Check sheet for the modelled part. Datum: model origin and axes. Units: mm. Face numbers are marked on the shaded views. A direction names the side the tool comes from. Give positions to 0.01 mm unless a question says otherwise; leave off trailing zeros. Order: outer loops, then holes, each group sorted by start corner. A loop starts at its lowest first (then second) coordinate and runs counter-clockwise, first axis right, second up.
Item 1: Access from +Z, -Z, +X, -X, +Y, -Y to the whole of each face (thin tool, end or side, straight path). Record for the marked faces 1, 2, 3 and 4.
Item 2: Gauge pin test, flat ends, axial feed: P1, Ø4, axis at x = -9, z = 12, coming from the +Y side; P2, Ø1.5, axis at x = 48, y = 7, coming from the +Z side; P3, Ø13, axis at x = -1, z = 28.5, coming from the -Y side. Record the tip position at first contact, or that the pin passes through.
Item 3: Material ranges on line 1 along Z through (x, y) = (-49.05, 13); line 2 along X through (y, z) = (19, 18); line 3 along Y through (x, z) = (-14.5, 10), recorded low to high.
Item 4: Sectioned sample at D-D on y = 6. Record the boundary of the cut face in (x, z).
Item 5: Sectioned sample at A-A on y = 13. Record the boundary of the cut face in (x, z).
Item 6: Sectioned sample at B-B on z = 23. Record the boundary of the cut face in (x, y), and give its area (3 significant figures).
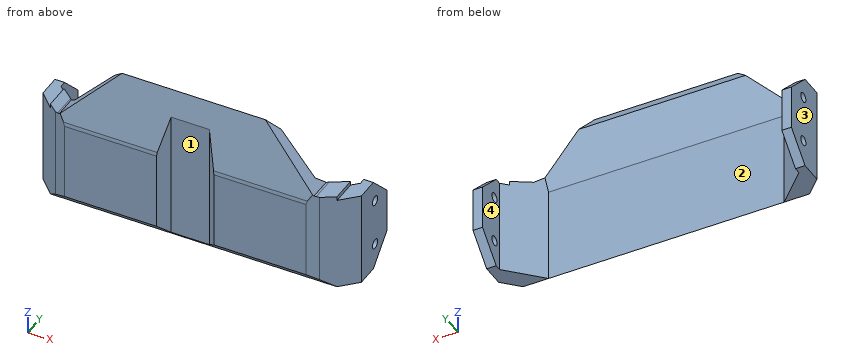
from build123d import *

# Parameters (mm, degrees)
F1_DEPTH      = 30
F2_SIZE       = 10
F4_DEPTH      = 50
F5_DEPTH      = 20
F6_DEPTH      = 25
F8_DEPTH      = 25.001
F9_DEPTH      = 25
F11_W         = 8
F11_H         = 3
F12_DEPTH     = 50.001
F13_T1_DEPTH  = 61.7168298797
F13_T3_DEPTH  = 40.0719817161
F13_T5_DEPTH  = 45.2357066129
F13_T10_DEPTH = 64.7177203375
F13_T15_DEPTH = 64.7177203375
F14_T1_DEPTH  = 56.7168298797
F14_T3_DEPTH  = 45.2357066129
F14_T5_DEPTH  = 35.0719817161
F15_R         = 1.5
F16_DEPTH     = 100.001
F18_SIZE      = 8
F19_SIZE      = 2.99999


# Not quite as in the source:
# - a fillet or chamfer that OpenCascade refuses, or shapes differently, is made with other operations: its cross-section is extruded or revolved along the edge and cut away or added
# - a fillet or chamfer is up to 0.001 mm smaller than in the source, because OpenCascade refuses the exact size


with BuildPart() as f1:
    # F0 (on Top) → F1 (new body)
    with BuildSketch(Plane.XY):
        Polygon((-47, 20), (-50, 20), (-50, -5), (50, -5), (50, 20), (47, 20), (47, 0), (-47, 0), align=None)
    extrude(amount=F1_DEPTH)

    # F2
    f2_edges = [f1.edges().sort_by_distance(p)[0] for p in [
        (-47, 0, 15),
        (47, 0, 15),
        (-50, -5, 15),
        (50, -5, 15),
    ]]
    chamfer(f2_edges, length=F2_SIZE)

    # F3 (on Right) → F4 (join, symmetric)
    with BuildSketch(Plane.YZ):
        Polygon((-5, 30), (0, 30), (2.9104275004, 49.2723931249), (0, 50), align=None)
    extrude(amount=F4_DEPTH, both=True)

    # F5 (add): faces of the model
    f5_faces = [f1.faces().sort_by_distance(p)[0] for p in [
        (46.0427350427, 7.6495726496, 30),
        (-46.0427350427, 7.6495726496, 30),
    ]]
    extrude(f5_faces, amount=F5_DEPTH)

    # F6 (cut): faces of the model
    f6_faces = [f1.faces().sort_by_distance(p)[0] for p in [
        (46.1111111111, -2.7777777778, 30),
        (-46.1111111111, -2.7777777778, 30),
    ]]
    extrude(f6_faces, amount=-F6_DEPTH, mode=Mode.SUBTRACT)

    # F7 (on face) → F8 (cut, through all)
    with BuildSketch(Plane.XZ.offset(5)):
        Polygon((40.5882352941, 32.3529411765), (45, 50), (37, 50), (22.5, 50), (40, 32.5), align=None)
        Polygon((45, 31.25), (45, 50), (40.5882352941, 32.3529411765), align=None)
        Polygon((45, 50), (47.9104275004, 49.2723931249), (45.1819017188, 31.2045245703), (50, 30), (50, 50), align=None)
    extrude(amount=-F8_DEPTH, mode=Mode.SUBTRACT)

    # F9 (cut): a face of the model
    f9_faces = [f1.faces().sort_by_distance(p)[0] for p in [
        (46.0411372728, 0, 41.900989059),
    ]]
    extrude(f9_faces, amount=-F9_DEPTH, mode=Mode.SUBTRACT)

    # F10: F1 across plane


with BuildPart() as f1_1:
    add(f1.part)
    add(f1.part.mirror(Plane.YZ), mode=Mode.INTERSECT)

    # F11 (on face) → F12 (cut, through all)
    with BuildSketch(Plane(origin=(0, 0, 0), x_dir=(1, 0, 0), z_dir=(0, 0, -1))):
        with Locations((0, 3.5)):
            Rectangle(F11_W, F11_H)
    extrude(amount=-F12_DEPTH, mode=Mode.SUBTRACT)

    # F13: chamfer of 5 on 5 edges, made by hand

    # F13_s2 → F13_t1 (cut)
    with BuildSketch(Plane.YZ.offset(-52.8584149398)):
        Polygon((0, 0), (-5, 5), (-5, 0), align=None)
    extrude(amount=F13_T1_DEPTH, mode=Mode.SUBTRACT)

    # F13_s4 → F13_t3 (cut)
    with BuildSketch(Plane.YZ.offset(-42.0359908581)):
        Polygon((-5, 29.3844718719), (-4.8507125007, 30.5971499971), (-5, 30), align=None)
    extrude(amount=F13_T3_DEPTH, mode=Mode.SUBTRACT)

    # F13_s6 → F13_t5 (cut)
    with BuildSketch(Plane.XY.offset(-5.6428543011)):
        Polygon((-41.4644660941, -3.5355339059), (-37.9289321881, -5), (-40, -5), align=None)
    extrude(amount=F13_T5_DEPTH, mode=Mode.SUBTRACT)


with BuildPart() as f13_tool8:
    # F13_s9 → F13_t10 (new body)
    with BuildSketch(Plane.XY.offset(-12.8584149398)):
        Polygon((9, -5), (4, 0), (4, -5), align=None)
    extrude(amount=F13_T10_DEPTH)

    split(bisect_by=Plane.XZ.offset(2), keep=Keep.TOP)


with BuildPart() as f1_2:
    add(f1_1.part)

    # F13_t7: cut F13_tool8
    add(f13_tool8.part, mode=Mode.SUBTRACT)


with BuildPart() as f13_tool13:
    # F13_s14 → F13_t15 (new body)
    with BuildSketch(Plane.XY.offset(-12.8584149398)):
        Polygon((-4, 0), (-9, -5), (-4, -5), align=None)
    extrude(amount=F13_T15_DEPTH)

    split(bisect_by=Plane.XZ.offset(2), keep=Keep.TOP)


with BuildPart() as f1_3:
    add(f1_2.part)

    # F13_t12: cut F13_tool13
    add(f13_tool13.part, mode=Mode.SUBTRACT)

    # F14: chamfer of 5 on 3 edges, made by hand

    # F14_s2 → F14_t1 (cut)
    with BuildSketch(Plane.YZ.offset(-3.8584149398)):
        Polygon((-5, 5), (0, 0), (-5, 0), align=None)
    extrude(amount=F14_T1_DEPTH, mode=Mode.SUBTRACT)

    # F14_s4 → F14_t3 (cut)
    with BuildSketch(Plane.XY.offset(-5.6428543011)):
        Polygon((41.4644660941, -3.5355339059), (37.9289321881, -5), (40, -5), align=None)
    extrude(amount=F14_T3_DEPTH, mode=Mode.SUBTRACT)

    # F14_s6 → F14_t5 (cut)
    with BuildSketch(Plane.YZ.offset(6.9640091419)):
        Polygon((-5, 29.3844718719), (-4.8507125007, 30.5971499971), (-5, 30), align=None)
    extrude(amount=F14_T5_DEPTH, mode=Mode.SUBTRACT)

    # F15 (on face) → F16 (cut, through all)
    with BuildSketch(Plane(origin=(-50, 0, 0), x_dir=(0, -1, 0), z_dir=(-1, 0, 0))):
        with Locations((-13, 23)):
            Circle(F15_R)
        with Locations((-13, 8)):
            Circle(F15_R)
    extrude(amount=-F16_DEPTH, mode=Mode.SUBTRACT)

    # F17: F1 across plane


with BuildPart() as f1_4:
    add(f1_3.part)
    add(f1_3.part.mirror(Plane.YZ), mode=Mode.INTERSECT)

    # F18
    f18_edges = [f1_4.edges().sort_by_distance(p)[0] for p in [
        (48.5, 20, 0),
        (-48.5, 20, 0),
        (-48.5, 20, 30),
        (48.5, 20, 30),
    ]]
    chamfer(f18_edges, length=F18_SIZE)

    # F19 (size 3 in the source; OpenCascade refuses exactly that, so slightly less here)
    f19_edges = [f1_4.edges().sort_by_distance(p)[0] for p in [
        (0, 2.910428, 49.272393),
    ]]
    chamfer(f19_edges, length=F19_SIZE)


solid = f1_4.part
Report:
1. face 1: +Z, -Z, -Y
1. face 2: -Z, +Y
1. face 3: +Z, -Z, -X, +Y, -Y
1. face 4: +Z, -Z, +Y
2. P1: stops at y = 0
2. P2: stops at z = 30
2. P3: stops at y = -3.5
3. line 1: z = 1 to 6.5, 9.5 to 21.5, 24.5 to 29
3. line 2: x = -50 to -47, 47 to 50
3. line 3: y = -5 to 0
4. outline: (-50, 0) - (-43, 0) - (-43, 31.75) - (-45, 31.25) - (-45, 30) - (-50, 30) - close; (43, 0) - (50, 0) - (50, 30) - (45, 30) - (45, 31.25) - (43, 31.75) - close
5. outline: (-50, 1) - (-47, 1) - (-47, 6.5) - (-50, 6.5) - close; (-50, 9.5) - (-47, 9.5) - (-47, 21.5) - (-50, 21.5) - close; (-50, 24.5) - (-47, 24.5) - (-47, 29) - (-50, 29) - close; (47, 1) - (50, 1) - (50, 6.5) - (47, 6.5) - close; (47, 9.5) - (50, 9.5) - (50, 21.5) - (47, 21.5) - close; (47, 24.5) - (50, 24.5) - (50, 29) - (47, 29) - close
6. outline: (-50, 5) - (-41.46, -3.54) - (-37.93, -5) - (-9, -5) - (-6, -2) - (6, -2) - (9, -5) - (37.93, -5) - (41.46, -3.54) - (50, 5) - (50, 11.5) - (47, 11.5) - (47, 10) - (37, 0) - (-37, 0) - (-47, 10) - (-47, 11.5) - (-50, 11.5) - close; (-50, 14.5) - (-47, 14.5) - (-47, 19) - (-50, 19) - close; (47, 14.5) - (50, 14.5) - (50, 19) - (47, 19) - close
6. area: 548 mm2
